```python
from build123d import *

# Parameters (mm, degrees)
BOSS_EXTRUDE1_DEPTH        = 6
F_3_2_3_2_DIAMETER_HOLE1_D = 3.2


with BuildPart() as part:
    # Sketch1 → Boss-Extrude1 (new body)
    with BuildSketch(Plane(origin=(0, 0, 0), x_dir=(1, 0, 0), z_dir=(0, 1, 0))):
        with BuildLine():
            Line((10, 28.7), (10, 45.4))
            Line((10, 45.4), (0, 45.4))
            Line((0, 45.4), (0, 0))
            Line((0, 0), (10, 0))
            Line((10, 0), (10, 16.7))
            ThreePointArc((10, 16.7), (4, 22.7), (10, 28.7))
        make_face()
    extrude(amount=BOSS_EXTRUDE1_DEPTH)

    # Ø3.2 (3.2) Diameter Hole1 (through all)
    with Locations(Plane.ZY):
        with Locations((-6, 3), (-39.4, 3)):
            Hole(F_3_2_3_2_DIAMETER_HOLE1_D / 2)


solid = part.part
```
Verification items for the finished model (mm, model axes). Round coordinates to 2 decimals unless told otherwise and drop trailing zeros. Order: outer loops, then holes, each group sorted by start corner. A loop starts at its lowest first (then second) coordinate and runs counter-clockwise, first axis right, second up.
1) Cross-section at A-A, the plane z = -6. Record the cut outline in (x, y), plus the area to 3 significant figures.
Geometry says:
outline: (0, 0) - (10, 0) - (10, 1.4) - (0, 1.4) - close; (0, 4.6) - (10, 4.6) - (10, 6) - (0, 6) - close
area: 28.0 mm2
2) Cross-section at B-B, the plane x = 9.25. Record the cut outline in (y, z).
Geometry says:
outline: (0, -45.4) - (6, -45.4) - (6, -28.65) - (0, -28.65) - close; (0, -16.75) - (6, -16.75) - (6, 0) - (0, 0) - close; hole circle Ø3.2 at (3, -39.4); hole circle Ø3.2 at (3, -6)
3) Cross-section at D-D, the plane y = 5.1. Record the cut outline in (x, z).
Geometry says:
outline: (0, -45.4) - (10, -45.4) - (10, -28.7) arc R6 cw to (10, -16.7) - (10, 0) - (0, 0) - close
4) Material ranges on line 1 (Y direction, x = 3.5, z = -6); line 2 (Z direction, x = 8.5, y = 3.35); line 3 (Z direction, x = 3.25, y = 2.9), recorded low to high.
Geometry says:
line 1: y = 0 to 1.4, 4.6 to 6
line 2: z = -45.4 to -40.96, -37.84 to -28.51, -16.89 to -7.56, -4.44 to 0
line 3: z = -45.4 to -41, -37.8 to -7.6, -4.4 to 0
5) Cross-section at C-C, the plane y = 2.25. Record the cut outline in (x, z), plus the area to 3 significant figures.
Geometry says:
outline: (0, -45.4) - (10, -45.4) - (10, -40.81) - (0, -40.81) - close; (0, -37.99) - (10, -37.99) - (10, -28.7) arc R6 cw to (10, -16.7) - (10, -7.41) - (0, -7.41) - close; (0, -4.59) - (10, -4.59) - (10, 0) - (0, 0) - close
area: 341 mm2
